```python
from build123d import *

# Parameters (mm, degrees)
BOSS_EXTRUDE1_DEPTH   = 3
SKETCH3_W             = 190.5
SKETCH3_H             = 25.4
BOSS_EXTRUDE2_DEPTH   = 3
BODY_MOVE_COPY1_ANGLE = 180
SKETCH5_W             = 25.4
SKETCH5_H             = 38.1
BOSS_EXTRUDE3_DEPTH   = 3
FILLET1_R             = 127
FILLET2_R             = 6.35
FILLET3_R             = 2.54
F_8_CLEARANCE_HOLE1_D = 4.4958


with BuildPart() as part:
    # Sketch1 → Boss-Extrude1 (new body)
    with BuildSketch(Plane.XY):
        Polygon((-381, 127), (0, 0), (0, 76.2), (-381, 203.2), align=None)
    extrude(amount=BOSS_EXTRUDE1_DEPTH)

    # Sketch3 → Boss-Extrude2 (add)
    with BuildSketch(Plane.XY.offset(3)):
        with Locations((-95.25, 12.7)):
            Rectangle(SKETCH3_W, SKETCH3_H)
    extrude(amount=-BOSS_EXTRUDE2_DEPTH)


with BuildPart() as body_2:
    # Body-Move_Copy1: copy of part
    add(part.part.rotate(Axis((-190.5, 0, 1.5), (0, 1, 0)), BODY_MOVE_COPY1_ANGLE))

    # Combine1: union part
    add(part.part)

    # Sketch5 → Boss-Extrude3 (add)
    with BuildSketch(Plane.XY.offset(3)):
        with Locations((-190.5, 44.45)):
            Rectangle(SKETCH5_W, SKETCH5_H)
    extrude(amount=-BOSS_EXTRUDE3_DEPTH)

    # Fillet1
    fillet1_edges = [body_2.edges().sort_by_distance(p)[0] for p in [
        (-190.5, 139.7, 1.5),
    ]]
    fillet(fillet1_edges, radius=FILLET1_R)

    # Fillet2
    fillet2_edges = [body_2.edges().sort_by_distance(p)[0] for p in [
        (-304.8, 101.6, 1.5),
        (-76.2, 101.6, 1.5),
        (-177.8, 59.266666667, 1.5),
        (-203.2, 25.4, 1.5),
        (-177.8, 25.4, 1.5),
        (-203.2, 59.266666667, 1.5),
    ]]
    fillet(fillet2_edges, radius=FILLET2_R)

    # Fillet3
    fillet3_edges = [body_2.edges().sort_by_distance(p)[0] for p in [
        (-304.8, 25.4, 1.5),
        (-76.2, 25.4, 1.5),
    ]]
    fillet(fillet3_edges, radius=FILLET3_R)

    # 8 Clearance Hole1 (through all)
    with Locations(Plane(origin=(0, 0, 0), x_dir=(-1, 0, 0), z_dir=(0, 0, -1))):
        with Locations((20.6375, 165.1), (360.3625, 165.1), (20.6375, 38.1), (360.3625, 38.1)):
            Hole(F_8_CLEARANCE_HOLE1_D / 2)


solid = body_2.part
```
Geometry check sheet. Reference: the model listing, model coordinates, mm. A direction names the side the tool comes from. Coordinates: 2 decimals unless noted, no trailing zeros. Loops run counter-clockwise (first coordinate to the right, second up) from the corner with the lowest first, then second, coordinate; pieces in that order, holes last. Notation, with made-up numbers: (-14, -11.5) -> (5, -11.5) arc R24 ccw to (5, 21.5) -> close; hole circle Ø2 at (-28.5, 46.5). An arc over 180 degrees is marked (long way). Put each result on its own line as item: value.
1) Tool access check on faces 4 (the flat face through (-130.8, 43.6, 1.5)), 5 (the flat face through (-76.2, 177.8, 1.5)), 6 (the flat face through (-352.343, 85.752, 1.521)). Record the directions out of +Z, -Z, +X, -X, +Y, -Y that give a thin tool (end or side, any length) a straight path to the whole face; none if there is none.
Result set:
face 4: +Z, -Z
face 5: +Z, -Z, +Y
face 6: +Z, -Z, -X
2) Cross-section at D-D on x = -270.5. Record the boundary of the cut face in (y, z), plus the area to 3 significant figures.
Result set:
outline: (0, 0) -> (25.4, 0) -> (25.4, 3) -> (0, 3) -> close; (36.83, 0) -> (166.37, 0) -> (166.37, 3) -> (36.83, 3) -> close
area: 465 mm^2
3) Gauge pin test, flat ends, axial feed: pin 1 Ø3.5 at (x, y) = (-360.36, 38.1) entering from +Z; pin 2 Ø0.9 at (x, z) = (-265, 1) entering from +Y; pin 3 Ø1.5 at (x, z) = (-142.5, 2) entering from +Y. Record the tip position at first contact, or that the pin passes through.
Result set:
pin 1: passes through
pin 2: stops at y = 164.68
pin 3: stops at y = 155.95
4) Cross-section at A-A on x = -42.5. Record the boundary of the cut face in (y, z).
Result set:
outline: (0, 0) -> (90.37, 0) -> (90.37, 3) -> (0, 3) -> close; (112.83, 0) -> (189.03, 0) -> (189.03, 3) -> (112.83, 3) -> close
5) Cross-section at C-C on y = 112. Record the boundary of the cut face in (x, z).
Result set:
outline: (-336, 0) -> (-45, 0) -> (-45, 3) -> (-336, 3) -> close
6) Cross-section at B-B on z = 2.5. Count the separate pieces of the cut face and the enclosed holes in it, plus the area to 3 significant figures.
Result set:
separate pieces: 1
enclosed holes: 6
area: 58,400 mm^2
7) Thickness scan on line 1 (Y direction, x = -254, z = 0.6); line 2 (Y direction, x = -340, z = 1.15); line 3 (Y direction, x = -184, z = 0.8). Record the ranges inside material, lowest first.
Result set:
line 1: y = 0 to 25.4, 42.33 to 160.87
line 2: y = 0 to 89.87, 113.33 to 189.53
line 3: y = 0 to 146.74
8) Release check for a two-part mould opening along Y. For faces 1 (the flat face through (-193, 80, 3)), 2 (the cylindrical face through (-189.93, 146.57, 1.48)), 3 (the flat face through (-250.2, 43.6, 1.5)) record: released by +Y, released by -Y, zero draft, split by the parting line, or undercut.
Result set:
face 1: zero draft
face 2: released by +Y
face 3: undercut
